Could you check a few things on this model? Use its own coordinates, in mm. A direction names the side the tool comes from. Round coordinates to 2 decimals unless told otherwise and drop trailing zeros. Write each loop counter-clockwise with the first axis right and the second up, starting at its lowest first coordinate (ties: lowest second). Pieces come first, ordered by that corner, then holes. Notation, with made-up numbers: (51, 32) -> (64, 32) arc R20 ccw to (64, 71) -> close; hole circle Ø10 at (-10, -30). An arc over 180 degrees is marked (long way). Answer in a Markdown table with one row per item.
from build123d import *

# Parameters (mm, degrees)
SKETCH1_W           = 76.2
SKETCH1_H           = 50.8
BOSS_EXTRUDE1_DEPTH = 101.6
SKETCH2_R           = 5.25
CUT_EXTRUDE1_DEPTH  = 300
SKETCH3_W           = 76.2
SKETCH3_H           = 76.2
CUT_EXTRUDE2_DEPTH  = 5


with BuildPart() as part:
    # Sketch1 → Boss-Extrude1 (new body)
    with BuildSketch(Plane(origin=(0, 0, 0), x_dir=(1, 0, 0), z_dir=(0, 1, 0))):
        with Locations((38.1, 25.4)):
            Rectangle(SKETCH1_W, SKETCH1_H)
    extrude(amount=BOSS_EXTRUDE1_DEPTH)

    # Sketch2 → Cut-Extrude1 (cut)
    with BuildSketch(Plane.XY):
        with Locations((38, 63)):
            Circle(SKETCH2_R)
    extrude(amount=-CUT_EXTRUDE1_DEPTH, mode=Mode.SUBTRACT)

    # Sketch3 → Cut-Extrude2 (cut)
    with BuildSketch(Plane.XY):
        with Locations((38.1, 63.5)):
            Rectangle(SKETCH3_W, SKETCH3_H)
    extrude(amount=-CUT_EXTRUDE2_DEPTH, mode=Mode.SUBTRACT)


solid = part.part
1) Imagine slicing it at D-D, the plane z = -2.5. Please give me the cut outline in (x, y).
Findings:
| item | result |
|---|---|
| outline | (0, 0) -> (76.2, 0) -> (76.2, 25.4) -> (0, 25.4) -> close |
2) Please list where these lines run through material, in increasing order: line 1 (X direction, y = 63.5, z = -7); line 2 (Y direction, x = 38, z = -24); line 3 (Z direction, x = 48.5, y = 33).
Findings:
| item | result |
|---|---|
| line 1 | x = 0 to 32.77, 43.23 to 76.2 |
| line 2 | y = 0 to 57.75, 68.25 to 101.6 |
| line 3 | z = -50.8 to -5 |
3) For faces 1 (the face through (38, 25.4, -2)), 2 (the face through (38, 50, -50.8)), which set-ups out of +Z, -Z, +X, -X, +Y, -Y let a thin tool reach every point of the face, with its end or its side?
Findings:
| item | result |
|---|---|
| face 1 | +Z, +X, -X, +Y |
| face 2 | -Z, +X, -X, +Y, -Y |
4) Imagine slicing it at A-A, the plane x = 38. Please give me the cut outline in (y, z), plus the area to 3 significant figures.
Findings:
| item | result |
|---|---|
| outline | (0, -50.8) -> (57.75, -50.8) -> (57.75, -5) -> (25.4, -5) -> (25.4, 0) -> (0, 0) -> close; (68.25, -50.8) -> (101.6, -50.8) -> (101.6, -5) -> (68.25, -5) -> close |
| area | 4,300 mm^2 |
5) For pin 1 (2.5 mm diameter, centred on x = 31, z = -1.5, fed in from +Y); pin 2 (13.5 mm diameter, centred on x = 38, y = 63, fed in from +Z), each with a flat end and sliding along its axis, tell me the tip position at first contact or that it passes through.
Findings:
| item | result |
|---|---|
| pin 1 | stops at y = 25.4 |
| pin 2 | stops at z = -5 |
6) Imagine slicing it at C-C, the plane x = 49. Please give me the cut outline in (y, z), plus the area to 3 significant figures.
Findings:
| item | result |
|---|---|
| outline | (0, -50.8) -> (101.6, -50.8) -> (101.6, -5) -> (25.4, -5) -> (25.4, 0) -> (0, 0) -> close |
| area | 4,780 mm^2 |
7) Imagine slicing it at B-B, the plane y = 63. Please give me the cut outline in (x, z).
Findings:
| item | result |
|---|---|
| outline | (0, -50.8) -> (32.75, -50.8) -> (32.75, -5) -> (0, -5) -> close; (43.25, -50.8) -> (76.2, -50.8) -> (76.2, -5) -> (43.25, -5) -> close |
8) Thinking about a two-plate mould opening in X: for faces 3 (the face through (76.2, 50, -25)), 4 (the face through (38, 13, 0)), 5 (the face through (36.862, 57.875, -27.579)), which applies, +X half, -X half, draft (parallel to the pull), parting line (faces both ways), or undercut?
Findings:
| item | result |
|---|---|
| face 3 | +X half |
| face 4 | draft |
| face 5 | undercut |
